Solid Edge part; units mm, degrees
sketch "Sketch1" plane through (0, 0, 0) normal (0, 0, 1) x (1, 0, 0)
  line L0 (-22, -9) -> (22, -9)
  line L1 (22, -9) -> (22, 9)
  line L2 (22, 9) -> (-22, 9)
  line L3 (-22, 9) -> (-22, -9)
extrude "Protrusion1" add sketch "Sketch1" along normal blind 3
sketch "Sketch2" plane through (0, 0, 3) normal (0, 0, 1) x (1, 0, 0)
  line L0 (24, -4) -> (14, -4)
  line L1 (14, -4) -> (14, 4)
  line L2 (14, 4) -> (24, 4)
  line L3 (24, 4) -> (24, -4)
extrude "ExtrudedProtrusion_2" add sketch "Sketch2" along normal blind 4
sketch "Sketch3" plane through (0, 0, 3) normal (0, 0, 1) x (1, 0, 0)
  line L0 (-22, -9) -> (22, -9)
  line L1 (22, -9) -> (22, -6)
  line L2 (22, -6) -> (-22, -6)
  line L3 (-22, -6) -> (-22, -9)
  line L4 (22, 6) -> (-22, 6)
  line L5 (-22, 6) -> (-22, 9)
  line L6 (-22, 9) -> (22, 9)
  line L7 (22, 9) -> (22, 6)
extrude "ExtrudedProtrusion_4" add sketch "Sketch3" along normal blind 9
Check sheet for the modelled part. Datum: model origin and axes. Units: mm. A direction names the side the tool comes from. Round coordinates to 2 decimals unless told otherwise and drop trailing zeros. Order: outer loops, then holes, each group sorted by start corner. A loop starts at its lowest first (then second) coordinate and runs counter-clockwise, first axis right, second up. Notation, with made-up numbers: (58, 16) - (82, 16) arc R22 ccw to (82, 51) - close; hole circle Ø9 at (-22, 32). An arc over 180 degrees is marked (long way). Write item = value, one per line.
Q1. Section check D-D (z = 9.25). Record the boundary of the cut face in (x, y).
Computed:
outline = (-22, -9) - (22, -9) - (22, -6) - (-22, -6) - close; (-22, 6) - (22, 6) - (22, 9) - (-22, 9) - close
Q2. Thickness scan on line 1 along Y through (x, z) = (18, 4.25); line 2 along Y through (x, z) = (-2.5, 3.25); line 3 along X through (y, z) = (-2.5, 1.5). Record the ranges inside material, lowest first.
Computed:
line_1 = -9 to -6, -4 to 4, 6 to 9
line_2 = -9 to -6, 6 to 9
line_3 = -22 to 22
Q3. Go/stop test with flat-tipped pins: pin 1 (4.5 mm diameter, centred on y = 1.5, z = 6, fed in from -X); pin 2 (5 mm diameter, centred on x = 7.5, y = -1, fed in from -Z); pin 3 (2 mm diameter, centred on x = -12.5, y = -3.5, fed in from +Z); pin 4 (1 mm diameter, centred on x = 23, y = 1.5, fed in from -Z). Record where each tip stops, or that it passes through.
Computed:
pin_1 = 14
pin_2 = 0
pin_3 = 3
pin_4 = 3
Q4. Section check B-B (y = -0.5). Record the boundary of the cut face in (x, z), and give its area (3 significant figures).
Computed:
outline = (-22, 0) - (22, 0) - (22, 3) - (24, 3) - (24, 7) - (14, 7) - (14, 3) - (-22, 3) - close
area = 172 mm^2
Q5. Draft check along Y on faces 1 (the face through (0, 9, 6)), 2 (the face through (0, -6, 7)), 3 (the face through (22, -2, 2)), 4 (the face through (0, -9, 6)). Enter one of: pulls with the +Y half, pulls with the -Y half, needs draft (parallel to the pull), parting line crosses it, or undercut.
Computed:
face_1 = pulls with the +Y half
face_2 = undercut
face_3 = needs draft
face_4 = pulls with the -Y half
Q6. Section check A-A (z = 6.5). Record the boundary of the cut face in (x, y), and give its area (3 significant figures).
Computed:
outline = (-22, -9) - (22, -9) - (22, -6) - (-22, -6) - close; (-22, 6) - (22, 6) - (22, 9) - (-22, 9) - close; (14, -4) - (24, -4) - (24, 4) - (14, 4) - close
area = 344 mm^2
Q7. Section check C-C (x = 18.5). Record the boundary of the cut face in (y, z), and give its area (3 significant figures).
Computed:
outline = (-9, 0) - (9, 0) - (9, 12) - (6, 12) - (6, 3) - (4, 3) - (4, 7) - (-4, 7) - (-4, 3) - (-6, 3) - (-6, 12) - (-9, 12) - close
area = 140 mm^2
Q8. Tool access check on faces 5 (the face through (14, 0, 5)), 6 (the face through (19, 0, 7)), 7 (the face through (-22, 2, 2)), 8 (the face through (23, 0, 3)), 9 (the face through (0, 0, 0)). Record the directions out of +Z, -Z, +X, -X, +Y, -Y that give a thin tool (end or side, any length) a straight path to the whole face; none if there is none.
Computed:
face_5 = +Z, -X
face_6 = +Z, +X, -X
face_7 = +Z, -Z, -X, +Y, -Y
face_8 = -Z, +X, +Y, -Y
face_9 = -Z, +X, -X, +Y, -Y
